Can you work these out from the model? Positions are in its coordinate system, mm. A direction names the side the tool comes from. Coordinates: 2 decimals unless noted, no trailing zeros. Order: outer loops, then holes, each group sorted by start corner. A loop starts at its lowest first (then second) coordinate and runs counter-clockwise, first axis right, second up. Notation, with made-up numbers: M 29,-10 L 38,-10 A24 cw 38,20 Z; hole C 4,66 d6. An arc over 180 degrees is marked long. Answer as CSV lines item,"result". Start each with the question number.
1. If we mould it in two halves opening along X, with no side actions, what happens to faces 4 (the face through (5, 0, 5)), 5 (the face through (4, 12, 1.3)), 6 (the face through (-4.864, -1.365, -4.461))? For each: released by +X, released by -X, zero draft, split by the parting line, or undercut.
2. If we section it at B-B (x = 0): List the corners of the cut face in (y, z) for me, plus the area to 3 significant figures.
3. I need wall thicknesses on line 1 along Z through (x, y) = (0, 12.9); line 2 along Z through (x, y) = (0, -1.5); line 3 along Y through (x, z) = (9.5, -6.75). Which ranges of each line are inside material? Lowest first, please. Write a range as from..to.
4. On a 3-axis mill with a long thin cutter (end or side, diameter ignored), from which of +Z, -Z, +X, -X, +Y, -Y can I reach the whole of each face in a straight line? I mean faces 1 (the face through (3.704, 5.908, -1.166)), 2 (the face through (-0.867, 12.625, -3.905)), 3 (the face through (5.2, 15, -0.2)). Say none if no direction works.
5. If we section it at A-A (z = 0): List the corners of the cut face in (x, y) for me.
6. If we section it at D-D (x = 7.25): List the corners of the cut face in (y, z) for me.
7. Will these pins go through, and if not, where does the flat tip stop? pin 1 (1.5 mm diameter, centred on x = -7.5, y = 9, fed in from +Z); pin 2 (2 mm diameter, centred on y = -2, z = -9, fed in from +X); pin 3 (6 mm diameter, centred on y = 11.5, z = -6, fed in from -X); pin 4 (1 mm diameter, centred on y = 8, z = 7, fed in from +X).
8. If we section it at C-C (y = 5): List the corners of the cut face in (x, z) for me, plus the area to 3 significant figures.
Autodesk Fusion 360 part; units mm, degrees
sketch "Sketch2" plane through (0, 0, 0) normal (0, 0, 1) x (1, 0, 0)
  line L0 (12, 15) -> (12, 0)
  line L1 (12, 0) -> (6.6, 0)
  line L2 (0, 0) -> (0, 15) construction
  line L3 (0, 15) -> (4, 15) construction
  line L4 (4, 15) -> (12, 15)
  line L5 (0, 0) -> (0, -4.5) construction
  line L6 (3, -4.5) -> (6.6, -4.5)
  line L7 (6.6, -4.5) -> (6.6, 0)
  line L8 (6.6, 0) -> (0, 0) construction
  line L9 (4, 15) -> (4, 12)
  line L10 (4, 12) -> (6.1, 12)
  line L11 (6.1, 12) -> (3, 3.4828)
  line L12 (3, 3.4828) -> (3, -4.5)
  line L13 (0, -4.5) -> (3, -4.5) construction
  dimension "d15" = 12
  dimension "d17" = 15
  dimension "d18" = 6.6
  dimension "d19" = 4
  dimension "d20" = 3
  dimension "d21" = 6.1
  dimension "d22" = 70
  dimension "d23" = 3
  dimension "d24" = 4.5
revolve "Revolve1" add sketch "Sketch2" angle 360 about axis through (0, 0, 0) along (0, 1, 0)
chamfer "Chamfer1" distance 1 angle 60 2 edges at (-3.7293, 15, -1.4465) (-6.1534, -4.5, -2.3867) measured on face at (9.2887, 15, 0.5962) measured on face at (5.3754, -4.5, 0.3279)
Solved:
1,face 4,"zero draft"
1,face 5,"undercut"
1,face 6,"split by the parting line"
2,outline,"M -4.5,-5.6 L -2.77,-6.6 L 0,-6.6 L 0,-12 L 15,-12 L 15,-5 L 13.27,-4 L 12,-4 L 12,-6.1 L 3.48,-3 L -4.5,-3 Z; M -4.5,3 L 3.48,3 L 12,6.1 L 12,4 L 13.27,4 L 15,5 L 15,12 L 0,12 L 0,6.6 L -2.77,6.6 L -4.5,5.6 Z"
2,area,"267 mm²"
3,line 1,"-12..-4, 4..12"
3,line 2,"-6.6..-3, 3..6.6"
3,line 3,"0..15"
4,face 1,"none"
4,face 2,"+Y"
4,face 3,"+Z, -Z, +X, -X, +Y"
5,outline,"M -12,0 L -6.6,0 L -6.6,-2.77 L -5.6,-4.5 L -3,-4.5 L -3,3.48 L -6.1,12 L -4,12 L -4,13.27 L -5,15 L -12,15 Z; M 3,-4.5 L 5.6,-4.5 L 6.6,-2.77 L 6.6,0 L 12,0 L 12,15 L 5,15 L 4,13.27 L 4,12 L 6.1,12 L 3,3.48 Z"
6,outline,"M 0,-9.56 L 15,-9.56 L 15,9.56 L 0,9.56 Z"
7,pin 1,"z = 9.92"
7,pin 2,"through"
7,pin 3,"x = -11.62"
7,pin 4,"x = 10.09"
8,outline,"C 0,0 d24; hole C 0,0 d7.1"
8,area,"413 mm²"
